Geometry check sheet. Reference: drawing and pictorial views, mm from the part's lowest x, y, z. A direction names the side the tool comes from. Round coordinates to 2 decimals unless told otherwise and drop trailing zeros. Order: outer loops, then holes, each group sorted by start corner. A loop starts at its lowest first (then second) coordinate and runs counter-clockwise, first axis right, second up.
Q1. Depth check by flat-ended pin: P1, Ø4, axis at y = 10.5, z = 43, coming from the -X side; P2, Ø8.5, axis at x = 6, y = 32, coming from the +Z side; P3, Ø1, axis at y = 10, z = 17, coming from the +X side; P4, Ø4, axis at x = 65.5, z = 23, coming from the -Y side. Enter the tip coordinate at first touch or a pass-through.
Q2. Cross-section at A-A on z = 19.05. Record the cut outline in (x, y), then the cut area to 3 significant figures.
Q3. Cross-section at B-B on x = 95.25. Record the cut outline in (y, z).
Q4. Set-up check for the marked faces 4 and 5: record each of +Z, -Z, +X, -X, +Y, -Y from which the full face is reachable in a straight line by a thin tool's end or side.
Q5. Cross-section at D-D on z = 4. Record the cut outline in (x, y), then the cut area to 3 significant figures.
Q6. Scan lines: probe 1 along X at (y, z) = (51, 19); probe 2 along Y at (x, z) = (33, 51.5); probe 3 along Z at (x, y) = (95.25, 48.75). Record each from-to range of solid material in increasing order.
Q7. Mould release check, pull along X, two halves, no side actions. Record for the marked faces 1, 2 and 3: +X half, -X half, draft (parallel to the pull), parting line (faces both ways), or undercut.
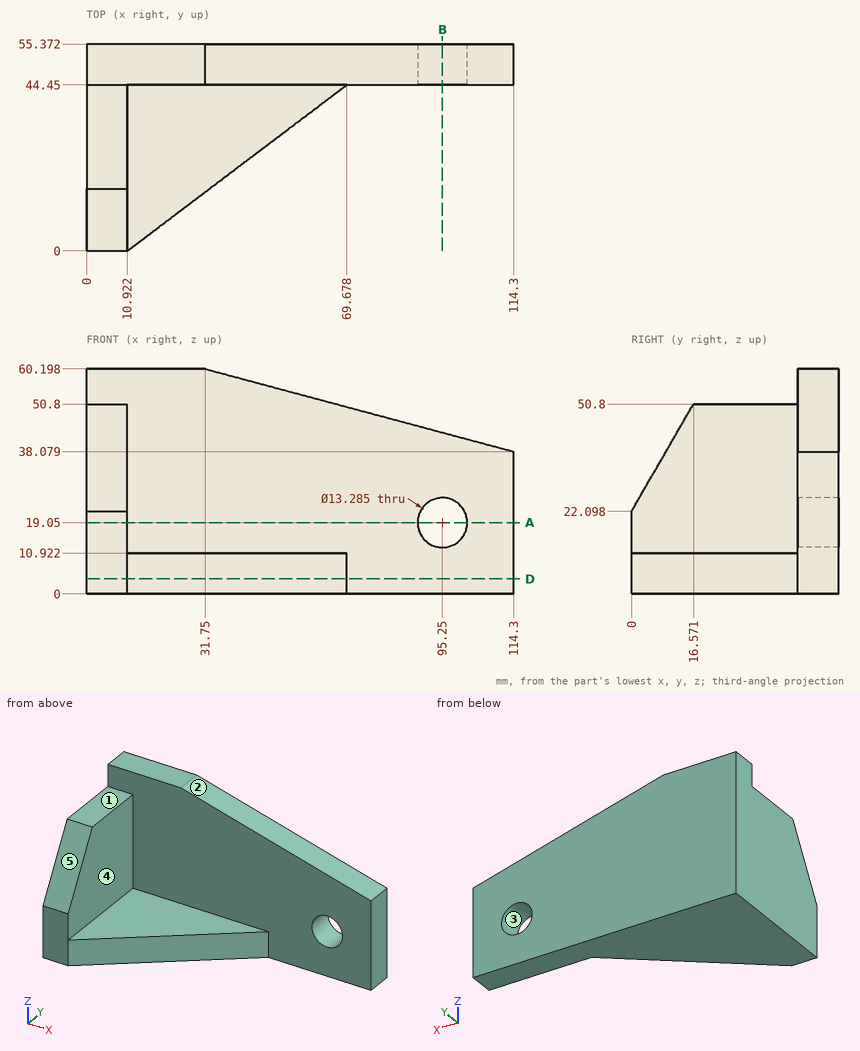
Results found:
1. P1: stops at x = 0
1. P2: stops at z = 50.8
1. P3: stops at x = 10.92
1. P4: stops at y = 44.45
2. outline: (0, 0) - (10.92, 0) - (10.92, 44.45) - (88.61, 44.45) - (88.61, 55.37) - (0, 55.37) - close; (101.89, 44.45) - (114.3, 44.45) - (114.3, 55.37) - (101.89, 55.37) - close
2. area: 1,590 mm2
3. outline: (44.45, 0) - (55.37, 0) - (55.37, 12.41) - (44.45, 12.41) - close; (44.45, 25.69) - (55.37, 25.69) - (55.37, 43.18) - (44.45, 43.18) - close
4. face 4: +Z, +X, -Y
4. face 5: +Z, +X, -X, -Y
5. outline: (0, 0) - (10.92, 0) - (69.68, 44.45) - (114.3, 44.45) - (114.3, 55.37) - (0, 55.37) - close
5. area: 3,040 mm2
6. probe 1: x = 0 to 88.61, 101.89 to 114.3
6. probe 2: y = 44.45 to 55.37
6. probe 3: z = 0 to 12.41, 25.69 to 43.18
7. face 1: draft
7. face 2: +X half
7. face 3: undercut
